Geometry check sheet. Reference: the model listing, model coordinates, mm. A direction names the side the tool comes from. Coordinates: 2 decimals unless noted, no trailing zeros. Loops run counter-clockwise (first coordinate to the right, second up) from the corner with the lowest first, then second, coordinate; pieces in that order, holes last. Notation, with made-up numbers: M -3,47.5 L 50,47.5 A32 ccw 50,74.5 Z; hole C 27,80 d3. An arc over 180 degrees is marked long. One line per question, with ' | ' between items. Start each with the question number.
from build123d import *

# Parameters (mm, degrees)
SKETCH1_R           = 23.999
SKETCH1_R_2         = 20.189
BOSS_EXTRUDE1_DEPTH = 12.7
SKETCH2_R           = 1.37499852
BOSS_EXTRUDE2_DEPTH = 3.81


with BuildPart() as part:
    # Sketch1 → Boss-Extrude1 (new body)
    with BuildSketch(Plane.XY):
        Circle(SKETCH1_R)
        Circle(SKETCH1_R_2, mode=Mode.SUBTRACT)
    extrude(amount=BOSS_EXTRUDE1_DEPTH)

    # Sketch2 → Boss-Extrude2 (add)
    with BuildSketch(Plane.XY.offset(12.7)):
        with BuildLine():
            Line((18.486532878, 15.303597719), (27.364357617, 25.428067959))
            ThreePointArc((27.364357617, 25.428067959), (27.970037037, 29.512520099), (24.499694037, 31.75))
            Line((24.499694037, 31.75), (-24.499694037, 31.75))
            ThreePointArc((-24.499694037, 31.75), (-27.970037037, 29.512520099), (-27.364357617, 25.428067959))
            Line((-27.364357617, 25.428067959), (-18.486532878, 15.303597719))
            ThreePointArc((-18.486532878, 15.303597719), (0, 23.999), (18.486532878, 15.303597719))
        make_face()
        with Locations((-24.499694037, 27.94)):
            Circle(SKETCH2_R, mode=Mode.SUBTRACT)
        with Locations((24.499694037, 27.94)):
            Circle(SKETCH2_R, mode=Mode.SUBTRACT)
    extrude(amount=-BOSS_EXTRUDE2_DEPTH)


solid = part.part
1. Sectioned sample at C-C (x = 0). Record the cut outline in (y, z).
2. Sectioned sample at A-A (y = 0). Record the cut outline in (x, z), and give its area (3 significant figures).
3. Draft check along Y on faces 1 (the flat face through (0, 31.75, 11)), 2 (the cylindrical face through (-24.8, 26.6, 10.8)), 3 (the flat face through (0, 25, 8.89)). Enter one of: +Y half, -Y half, draft (parallel to the pull), parting line (faces both ways), or undercut.
4. Thickness scan on line 1 (Y direction, x = 0, z = 7.5); line 2 (X direction, y = 29, z = 9); line 3 (X direction, y = -2, z = 10). Record the ranges inside material, lowest first.
5. Sectioned sample at D-D (y = 27.94). Record the cut outline in (x, z).
6. Sectioned sample at B-B (z = 11.5). Record the cut outline in (x, y) (3 decimals).
7. Tool access check on faces 4 (the flat face through (22.86, 20.29, 10.82)), 5 (the cylindrical face through (-5.2, -23.43, 6.26)), 6 (the flat face through (-22.99, 20.44, 10.82)). Record the directions out of +Z, -Z, +X, -X, +Y, -Y that give a thin tool (end or side, any length) a straight path to the whole face; none if there is none.
8. Depth check by flat-ended pin: pin 1 Ø1 at (x, z) = (12.5, 11) entering from -Y; pin 2 Ø3 at (x, y) = (-24.5, 27.94) entering from -Z; pin 3 Ø13 at (x, y) = (9.5, 21) entering from -Z; pin 4 Ø2 at (x, z) = (8, 4.5) entering from +Y. Enter the tip coordinate at first touch or a pass-through.
Result:
1) outline: M -24,0 L -20.19,0 L -20.19,12.7 L -24,12.7 Z; M 20.19,0 L 24,0 L 24,8.89 L 31.75,8.89 L 31.75,12.7 L 20.19,12.7 Z
2) outline: M -24,0 L -20.19,0 L -20.19,12.7 L -24,12.7 Z; M 20.19,0 L 24,0 L 24,12.7 L 20.19,12.7 Z | area: 96.8 mm2
3) face 1: +Y half | face 2: undercut | face 3: draft
4) line 1: y = -24 to -20.19, 20.19 to 24 | line 2: x = -28.16 to -25.38, -23.62 to 23.62, 25.38 to 28.16 | line 3: x = -23.92 to -20.09, 20.09 to 23.92
5) outline: M -28.31,8.89 L -25.87,8.89 L -25.87,12.7 L -28.31,12.7 Z; M -23.12,8.89 L 23.12,8.89 L 23.12,12.7 L -23.12,12.7 Z; M 25.87,8.89 L 28.31,8.89 L 28.31,12.7 L 25.87,12.7 Z
6) outline: M -27.364,25.428 L -18.487,15.304 A23.999 ccw long 18.487,15.304 L 27.364,25.428 A3.81 ccw 24.5,31.75 L -24.5,31.75 A3.81 ccw Z; hole C -24.5,27.94 d2.75; hole C 0,0 d40.378; hole C 24.5,27.94 d2.75
7) face 4: +Z, -Z, +X | face 5: -Z | face 6: +Z, -Z, -X
8) pin 1: stops at y = -20.78 | pin 2: stops at z = 8.89 | pin 3: stops at z = 0 | pin 4: stops at y = 22.96
